For this review, take the finished solid that the model builds, in its own axes (mm). A direction names the side the tool comes from. Round coordinates to 2 decimals unless told otherwise and drop trailing zeros. Order: outer loops, then holes, each group sorted by start corner. A loop starts at its lowest first (then second) coordinate and runs counter-clockwise, first axis right, second up. Notation, with made-up numbers: (68, 55.5) -> (100, 55.5) arc R20 cw to (100, 89.5) -> close; hole circle Ø2 at (84.25, 27). An arc over 180 degrees is marked (long way). Put each result on its own line as item: value. Start each with the question number.
```python
from build123d import *

# Parameters (mm, degrees)
BOSS_EXTRUDE1_DEPTH = 6
FILLET1_R           = 1


with BuildPart() as part:
    # Sketch1 → Boss-Extrude1 (new body)
    with BuildSketch(Plane(origin=(0, 0, 0), x_dir=(1, 0, 0), z_dir=(0, 1, 0))):
        Polygon((-29.75, 2.9), (29.75, 2.9), (29.75, 5.15), (32.15, 5.15), (32.15, -2.25), (29.75, -2.25), (29.75, 0), (-29.75, 0), (-29.75, -2.25), (-32.15, -2.25), (-32.15, 5.15), (-29.75, 5.15), align=None)
    extrude(amount=BOSS_EXTRUDE1_DEPTH)

    # Fillet1
    fillet1_edges = [part.edges().sort_by_distance(p)[0] for p in [
        (0, 0, -2.9),
        (29.75, 0, -4.025),
        (30.95, 0, -5.15),
        (32.15, 0, -1.45),
        (30.95, 0, 2.25),
        (29.75, 0, 1.125),
        (0, 0, 0),
        (-29.75, 0, 1.125),
        (-30.95, 0, 2.25),
        (-32.15, 0, -1.45),
        (-30.95, 0, -5.15),
        (-29.75, 0, -4.025),
    ]]
    fillet(fillet1_edges, radius=FILLET1_R)


solid = part.part
```
Item 1: Consider section C-C, the plane x = 24. Write out the cut boundary in (y, z).
Item 2: Consider section A-A, the plane z = -3.5. Write out the cut boundary in (x, y).
Item 3: Insertion check: pin 1 Ø1.5 at (x, y) = (20.5, 4) entering from +Z; pin 2 Ø3 at (x, y) = (20, 1.5) entering from -Z; pin 3 Ø1.5 at (x, z) = (-18.5, -4) entering from +Y. Each pin has a flat end and moves straight along its axis. Give the tip position at first contact, or say it passes through.
Item 4: Tool access review of faces 5 (the face through (-29.75, 3, -4)), 6 (the face through (-29.75, 3, 1)), 7 (the face through (30.035, 0.301, 0.602)), 8 (the face through (30.035, 0.301, -3.548)): name each direction out of +Z, -Z, +X, -X, +Y, -Y from which nothing blocks a thin tool from reaching the whole face with its end or side.
Item 5: Consider section B-B, the plane y = 3.05. Write out the cut boundary in (x, z), plus the area to 3 significant figures.
Item 6: For L1, parallel to X at y = 1.7, z = -3.5; L2, parallel to Z at x = -1.5, y = 4.55; L3, parallel to Y at x = -5.5, z = -2, list the stretches that pass through material, from the lowest coordinate up.
Item 7: Mouldability with a two-part tool opening along X and no side actions: class faces 1 (the face through (-30.035, 0.301, 0.648)), 2 (the face through (30.97, 0.44, -4.98)), 3 (the face through (-32.15, 3, -1)), 4 (the face through (0, 3, 0)) as +X half, -X half, draft (parallel to the pull), parting line (faces both ways), or undercut.
Evaluation:
1. outline: (0, -1.9) arc R1 ccw to (1, -2.9) -> (6, -2.9) -> (6, 0) -> (1, 0) arc R1 ccw to (0, -1) -> close
2. outline: (-32.15, 1) arc R1 ccw to (-31.15, 0) -> (-30.75, 0) arc R1 ccw to (-29.75, 1) -> (-29.75, 6) -> (-32.15, 6) -> close; (29.75, 1) arc R1 ccw to (30.75, 0) -> (31.15, 0) arc R1 ccw to (32.15, 1) -> (32.15, 6) -> (29.75, 6) -> close
3. pin 1: stops at z = 0
3. pin 2: stops at z = -2.9
3. pin 3: passes through
4. face 5: -Z, +Y, -Y
4. face 6: +Z, +Y, -Y
4. face 7: +Z, -Y
4. face 8: -Z, -Y
5. outline: (-32.15, -5.15) -> (-29.75, -5.15) -> (-29.75, -2.9) -> (29.75, -2.9) -> (29.75, -5.15) -> (32.15, -5.15) -> (32.15, 2.25) -> (29.75, 2.25) -> (29.75, 0) -> (-29.75, 0) -> (-29.75, 2.25) -> (-32.15, 2.25) -> close
5. area: 208 mm^2
6. L1: x = -32.15 to -29.75, 29.75 to 32.15
6. L2: z = -2.9 to 0
6. L3: y = 0.01 to 6
7. face 1: undercut
7. face 2: draft
7. face 3: -X half
7. face 4: undercut
